CAD build for the part. Positions are in the model's coordinates, mm. A direction names the side the tool comes from. Round coordinates to 2 decimals unless told otherwise and drop trailing zeros. Order: outer loops, then holes, each group sorted by start corner. A loop starts at its lowest first (then second) coordinate and runs counter-clockwise, first axis right, second up. Notation, with made-up numbers: (71, 33) - (104, 33) arc R23 ccw to (104, 62) - close; hole circle Ø1 at (-37.5, 22). An arc over 180 degrees is marked (long way). Write item = value, one per line.
Autodesk Inventor part; units mm, degrees
ref_plane "Work Plane1" through (0, 0, -17) normal (0, 0, -1) x (-1, 0, 0)
ref_plane "Work Plane2" through (0, 0, 29) normal (0, 0, 1) x (1, 0, 0)
ref_plane "YZ Plane" through (0, 0, 0) normal (1, 0, 0) x (0, 1, 0)
sketch "Sketch1" plane through (0, 0, 0) normal (0, 0, 1) x (1, 0, 0)
  circle A0 centre (0, 0) radius 4
  dimension "d0" = 8
extrude "Extrusion1" add sketch "Sketch1" along normal blind 54
sketch "Sketch2" plane through (0, 0, 0) normal (0, 0, -1) x (-1, 0, 0)
  line L0 (0, 7.5056) -> (6.5, 3.7528)
  line L1 (6.5, 3.7528) -> (6.5, -3.7528)
  line L2 (6.5, -3.7528) -> (0, -7.5056)
  line L3 (0, -7.5056) -> (-6.5, -3.7528)
  line L4 (-6.5, -3.7528) -> (-6.5, 3.7528)
  line L5 (-6.5, 3.7528) -> (0, 7.5056)
  point P0 (0, 0)
  point P1 (0, 0)
  dimension "d3" = 13
  dimension "d4" = 6.5
extrude "Extrusion2" add sketch "Sketch2" along normal blind 6
sketch "Sketch3" plane through (0, 0, -6) normal (0, 0, -1) x (-1, 0, 0)
  circle A0 centre (0, 0) radius 8.5
  dimension "d7" = 17
extrude "Extrusion3" add sketch "Sketch3" along normal blind 1
sketch "Sketch4" plane through (0, 0, -7) normal (0, 0, -1) x (-1, 0, 0)
  circle A0 centre (0, 0) radius 7.5
  dimension "d10" = 15
ref_plane "Work Plane1" through (0, 0, -17) normal (0, 0, -1) x (-1, 0, 0)
sketch "Sketch5" plane through (0, 0, -17) normal (0, 0, -1) x (-1, 0, 0)
  circle A0 centre (0, 0) radius 14.5
  dimension "d12" = 29
loft "Loft1" add profiles "Sketch4", "Sketch5"
sketch "Sketch6" plane through (0, 0, -17) normal (0, 0, -1) x (-1, 0, 0)
  circle A0 centre (0, 0) radius 17
  dimension "d17" = 34
extrude "Extrusion4" add sketch "Sketch6" against normal blind 2
chamfer "Chamfer1" distance 0.3 angle 45 1 edges at (-4, 0, 54)
sketch "Sketch7" plane through (0, 0, -17) normal (0, 0, -1) x (-1, 0, 0)
  circle A0 centre (0, 0) radius 4
  circle A1 centre (0, 0) radius 20
  dimension "d26" = 40
extrude "Extrusion5" add sketch "Sketch7" against normal blind 4 and the other way blind 5
sketch "Sketch8" plane through (0, 0, -22) normal (0, 0, -1) x (-1, 0, 0)
  circle A0 centre (0, 0) radius 8
  dimension "d31" = 16
extrude "Extrusion6" cut sketch "Sketch8" against normal blind 12
sketch "Sketch9" plane through (0, 0, 0) normal (0, 0, 1) x (1, 0, 0)
  line L0 (0, 7.5056) -> (-6.5, 3.7528)
  line L1 (-6.5, 3.7528) -> (-6.5, -3.7528)
  line L2 (-6.5, -3.7528) -> (0, -7.5056)
  line L3 (0, -7.5056) -> (6.5, -3.7528)
  line L4 (6.5, -3.7528) -> (6.5, 3.7528)
  line L5 (6.5, 3.7528) -> (0, 7.5056)
  circle A0 centre (0, 0) radius 4
extrude "Extrusion7" cut sketch "Sketch9" against normal up to surface (6 mm away)
ref_plane "Work Plane2" through (0, 0, 29) normal (0, 0, 1) x (1, 0, 0)
sketch "Sketch10" plane through (0, 0, 29) normal (0, 0, 1) x (1, 0, 0)
  circle A0 centre (0, 0) radius 4
  line L0 (8.6603, 0) -> (4.3301, -7.5)
  line L1 (4.3301, -7.5) -> (-4.3301, -7.5)
  line L2 (-4.3301, -7.5) -> (-8.6603, 0)
  line L3 (-8.6603, 0) -> (-4.3301, 7.5)
  line L4 (-4.3301, 7.5) -> (4.3301, 7.5)
  line L5 (4.3301, 7.5) -> (8.6603, 0)
  dimension "d37" = 15
  dimension "d38" = 8.6602
  dimension "d39" = 8.6602
extrude "Extrusion8" add sketch "Sketch10" against normal blind 5.5
thread "Thread2"
thread "Thread3"
equation "\"d4\" = 0.5 * d3"
properties part number "Adjuster Pad" material "Stainless Steel"
(1) Band-saw the part on C-C on z = -8. List the corners of the cut face in (x, y), plus the area to 3 significant figures.
Solved:
outline = circle Ø16.4 at (0, 0)
area = 211 mm²
(2) Pull direction Z, two halves, no side cores. Call faces 1 (the conical face through (-7.404, 2.332, -7.375)), 2 (the flat face through (0, -8, -7)), 3 (the flat face through (4, 2, 29)), 4 (the flat face through (0, 0, -10)): released by +Z, released by -Z, zero draft, split by the parting line, or undercut.
Solved:
face_1 = undercut
face_2 = undercut
face_3 = released by +Z
face_4 = released by -Z
(3) Tool access for faces 5 (the flat face through (-6.465, -3.802, 26.288)), 6 (the cylindrical face through (-0.867, 3.905, 8.544)), 7 (the flat face through (-9, -9, -13)), 8 (the cylindrical face through (1.73, -7.81, -16.08)): list every direction of +Z, -Z, +X, -X, +Y, -Y with a clear straight run to the whole face (end or side of a thin tool).
Solved:
face_5 = +Z, -X, -Y
face_6 = none
face_7 = +Z
face_8 = -Z
(4) Band-saw the part on D-D on z = 2. List the corners of the cut face in (x, y), plus the area to 3 significant figures.
Solved:
outline = circle Ø8 at (0, 0)
area = 50.3 mm²
(5) Drop flat-ended pins along their axis: pin 1 (1 mm diameter, centred on x = -6, z = 6, fed in from +Y); pin 2 (3 mm diameter, centred on x = -1.5, z = 26, fed in from -Y); pin 3 (4.5 mm diameter, centred on x = 0, y = -1.5, fed in from -Z); pin 4 (12 mm diameter, centred on x = 12, y = 5, fed in from +Z). Give the stop position or say it passes through.
Solved:
pin_1 = through
pin_2 = -7.5
pin_3 = -10
pin_4 = 29
(6) Probe line 1 along Y through (x, z) = (0, -16); line 2 along X through (y, z) = (-6, -11.5); line 3 along Z through (x, y) = (-13, -14). List the from-to ranges inside material, lowest first.
Solved:
line_1 = -20 to -8, 8 to 20
line_2 = -8.8 to -5.29, 5.29 to 8.8
line_3 = -22 to -13
(7) Band-saw the part on B-B on y = 16. List the corners of the cut face in (x, z).
Solved:
outline = (-12, -22) - (12, -22) - (12, -13) - (-12, -13) - close
